```python
from build123d import *

# Parameters (mm, degrees)
FILLET003_R = 2.6


with BuildPart() as railfillet:
    # Sweep: sweep along a path in Sketch002
    with BuildLine(Plane.XZ) as sweep_path:
        Line((6.5, 0), (6.5, 19))
        ThreePointArc((6.5, 19), (7.671582, 21.828411), (10.5, 22.999974))
        Line((10.5, 22.999974), (18.5, 22.999974))
    # Sketch011 → Sweep (sweep)
    with BuildSketch(Plane.XY):
        Polygon((10.2, 4.366273), (5.833727, 0), (10.2, -4.366273), align=None)
    sweep(path=sweep_path.line)

    # Fillet003
    fillet003_edges = [railfillet.edges().sort_by_distance(p)[0] for p in [
        (14.499996, -1.3e-05, 23.66626),
    ]]
    fillet(fillet003_edges, radius=FILLET003_R)


with BuildPart() as guide:
    # Part__Mirroring: instance of RailFillet
    add(railfillet.part.mirror(Plane(origin=(0, 0, 0), x_dir=(0, 1, 0), z_dir=(0, 0, 1))))

    # Fusion001: union RailFillet
    add(railfillet.part)


solid = guide.part
```
Source: CAD feature listing. Evaluate the final solid. Frame: model axes, mm. A direction names the side the tool comes from. Give positions to 0.01 mm unless a question says otherwise; leave off trailing zeros. Order: outer loops, then holes, each group sorted by start corner. A loop starts at its lowest first (then second) coordinate and runs counter-clockwise, first axis right, second up.
(1) Section query B-B (z = 7.5). Return the cut outline in (x, y).
(2) Pull-direction query (Z, two-part tool) for faces 1 (the face through (9.39, -3.12, -20.08)), 2 (the face through (10.2, 0, 0)), 3 (the face through (14.56, 0.03, 22.59)); classes: +Z half, -Z half, draft (parallel to the pull), parting line (faces both ways), or undercut.
(3) Section query A-A (y = 3.25). Return the cut outline in (x, z), plus the area to 3 significant figures.
(4) Section query C-C (y = -2.75). Return the cut outline in (x, z).
(5) Access query for faces 4 (the face through (15, 0, -19.3)), 5 (the face through (14.556, 3.12, 20.546)). Directions: +Z, -Z, +X, -X, +Y, -Y. A direction counts if a zero-diameter tool reaches every point of the face in a straight line with its end or side. Return the directions, or none.
(6) Contact query for flat-ended pins moving along their axis: P1, Ø3, axis at x = 17, z = 16.5, coming from the -Y side; P2, Ø6, axis at x = 12, z = -0.5, coming from the +Y side; P3, Ø3, axis at y = -3, z = -7.5, coming from the +X side; P4, Ø1, axis at x = 12.5, y = -1.5, coming from the -Z side. Output: stop coordinate, or through.
(7) Material intervals for line 1 along Z through (x, y) = (14, -0.5); line 2 along Z through (x, y) = (13.25, 1.75); line 3 along X through (y, z) = (0, 3), sorted ascending.
Outcome:
1. outline: (7.67, -1.84) - (10.2, -4.37) - (10.2, 4.37) - (7.67, 1.84) arc R2.6 ccw to start
2. face 1: -Z half
2. face 2: undercut
2. face 3: +Z half
3. outline: (9.08, -19) arc R1.42 ccw to (10.5, -20.42) - (18.5, -20.42) - (18.5, -19.3) - (10.5, -19.3) arc R0.3 cw to (10.2, -19) - (10.2, 19) arc R0.3 cw to (10.5, 19.3) - (18.5, 19.3) - (18.5, 20.42) - (10.5, 20.42) arc R1.42 ccw to (9.08, 19) - close
3. area: 63.3 mm2
4. outline: (8.58, -19) arc R1.92 ccw to (10.5, -20.92) - (18.5, -20.92) - (18.5, -19.3) - (10.5, -19.3) arc R0.3 cw to (10.2, -19) - (10.2, 19) arc R0.3 cw to (10.5, 19.3) - (18.5, 19.3) - (18.5, 20.92) - (10.5, 20.92) arc R1.92 ccw to (8.58, 19) - close
5. face 4: +X, +Y, -Y
5. face 5: +Z, +X, -X, +Y
6. P1: passes through
6. P2: stops at y = 4.37
6. P3: stops at x = 10.2
6. P4: stops at z = -22.39
7. line 1: z = -22.54 to -19.3, 19.3 to 22.54
7. line 2: z = -21.91 to -19.3, 19.3 to 21.91
7. line 3: x = 6.91 to 10.2
